from build123d import *

# Parameters (mm, degrees)
SKETCH1_W           = 90
SKETCH1_H           = 90
BOSS_EXTRUDE1_DEPTH = 3.1
SKETCH2_R           = 1.65
CUT_EXTRUDE1_DEPTH  = 128.316966662
SKETCH5_R           = 2.95
CUT_EXTRUDE2_DEPTH  = 2.5


with BuildPart() as part:
    # Sketch1 → Boss-Extrude1 (new body)
    with BuildSketch(Plane(origin=(0, 0, 0), x_dir=(1, 0, 0), z_dir=(0, 1, 0))):
        with Locations((45, 45)):
            Rectangle(SKETCH1_W, SKETCH1_H)
    extrude(amount=-BOSS_EXTRUDE1_DEPTH)

    # Sketch2 → Cut-Extrude1 (cut, through all)
    with BuildSketch(Plane.XZ.offset(3.1)):
        with Locations(Location((45, -42, 0), (0, 0, 270))):
            Circle(SKETCH2_R)
        with Locations(Location((45, -48, 0), (0, 0, 270))):
            Circle(SKETCH2_R)
    extrude(amount=-CUT_EXTRUDE1_DEPTH, mode=Mode.SUBTRACT)

    # Sketch5 → Cut-Extrude2 (cut)
    with BuildSketch(Plane.XZ.offset(3.1)):
        with Locations(Location((45, -42, 0), (0, 0, 270))):
            Circle(SKETCH5_R)
        with Locations(Location((45, -48, 0), (0, 0, 270))):
            Circle(SKETCH5_R)
    extrude(amount=-CUT_EXTRUDE2_DEPTH, mode=Mode.SUBTRACT)


solid = part.part
Source: CAD feature listing. Evaluate the final solid. Frame: model axes, mm. A direction names the side the tool comes from. Give positions to 0.01 mm unless a question says otherwise; leave off trailing zeros. Order: outer loops, then holes, each group sorted by start corner. A loop starts at its lowest first (then second) coordinate and runs counter-clockwise, first axis right, second up. Notation, with made-up numbers: (61, 32) -> (112, 32) arc R27 ccw to (112, 53) -> close; hole circle Ø2 at (78, 9.25). An arc over 180 degrees is marked (long way). Write item = value, one per line.
Q1. Pull-direction query (X, two-part tool) for faces 3 (the face through (0, -2, -44)), 4 (the face through (43.205, -1.868, -45.659)), 5 (the face through (90, -2, -44)), 6 (the face through (44, 0, -46)); classes: released by +X, released by -X, zero draft, split by the parting line, or undercut.
Data:
face_3 = released by -X
face_4 = undercut
face_5 = released by +X
face_6 = zero draft
Q2. Cut plane A-A, the plane x = 45. Output: boundary loops of the cut face in (y, z), and give its area (3 significant figures).
Data:
outline = (-3.1, -90) -> (0, -90) -> (0, -49.65) -> (-0.6, -49.65) -> (-0.6, -50.95) -> (-3.1, -50.95) -> close; (-3.1, -45.05) -> (-0.6, -45.05) -> (-0.6, -46.35) -> (0, -46.35) -> (0, -43.65) -> (-0.6, -43.65) -> (-0.6, -44.95) -> (-3.1, -44.95) -> close; (-3.1, -39.05) -> (-0.6, -39.05) -> (-0.6, -40.35) -> (0, -40.35) -> (0, 0) -> (-3.1, 0) -> close
area = 246 mm^2
Q3. Set-up query: faces 1 (the face through (43.7, -0.6, -49.3)), 2 (the face through (44, -2, 0)). Return all of +Z, -Z, +X, -X, +Y, -Y with unobstructed straight access to the full face (end or side cutting, diameter ignored); none if empty.
Data:
face_1 = -Y
face_2 = +Z, +X, -X, +Y, -Y
Q4. Pin query (flat end, axial travel): pin 1 (1.5 mm diameter, centred on x = 30, z = -71, fed in from +Y); pin 2 (4.5 mm diameter, centred on x = 45, z = -41.5, fed in from -Y). Return the tip coordinate at first contact, or that it passes through.
Data:
pin_1 = 0
pin_2 = -0.6
Q5. Material intervals for line 1 (X direction, y = -0.2, z = -48); line 2 (X direction, y = -1.6, z = -42), sorted ascending. Write a range as from..to.
Data:
line_1 = 0..43.35, 46.65..90
line_2 = 0..42.05, 47.95..90
Q6. Cut plane B-B, the plane z = -42. Output: boundary loops of the cut face in (x, y), and give its area (3 significant figures).
Data:
outline = (0, -3.1) -> (42.05, -3.1) -> (42.05, -0.6) -> (43.35, -0.6) -> (43.35, 0) -> (0, 0) -> close; (46.65, -0.6) -> (47.95, -0.6) -> (47.95, -3.1) -> (90, -3.1) -> (90, 0) -> (46.65, 0) -> close
area = 262 mm^2
